```python
from build123d import *

# Parameters (mm, degrees)
F0_R     = 6.35
F1_DEPTH = 12.7
F2_R     = 1.5875
F3_DEPTH = 10.16
F4_W     = 0.4064
F4_H     = 3.728392
F5_DEPTH = 11.4554
F6_SIZE  = 1.27


with BuildPart() as f1:
    # F0 (on Top) → F1 (new body)
    with BuildSketch(Plane.XY):
        Circle(F0_R)
    extrude(amount=-F1_DEPTH)

    # F2 (on face) → F3 (cut)
    with BuildSketch(Plane.XY):
        Circle(F2_R)
    extrude(amount=-F3_DEPTH, mode=Mode.SUBTRACT)

    # F4 (on Top) → F5 (join)
    with BuildSketch(Plane.XY):
        Rectangle(F4_W, F4_H)
    extrude(amount=-F5_DEPTH)

    # F6
    f6_edges = [f1.edges().sort_by_distance(p)[0] for p in [
        (-6.35, 0, -12.7),
    ]]
    chamfer(f6_edges, length=F6_SIZE)


solid = f1.part
```
The model under review builds one solid part; all positions refer to its coordinate system, in mm. A direction names the side the tool comes from. Give positions to 0.01 mm unless a question says otherwise; leave off trailing zeros. Loops run counter-clockwise (first coordinate to the right, second up) from the corner with the lowest first, then second, coordinate; pieces in that order, holes last. Notation, with made-up numbers: (31, -24.5) - (69, -24.5) arc R27 cw to (69, -6.5) - close; hole circle Ø7 at (-28, 67). An arc over 180 degrees is marked (long way). Answer as a JSON object with one key per item and string values.
Q1. Insertion check: pin 1 (3 mm diameter, centred on y = 0.5, z = -9, fed in from +X); pin 2 (1.5 mm diameter, centred on x = 2.5, z = -6, fed in from +Y); pin 3 (2 mm diameter, centred on x = 2.5, z = -9.5, fed in from +Y); pin 4 (2 mm diameter, centred on x = 3, z = -6.5, fed in from +Y). Each pin has a flat end and moves straight along its axis. Give the tip position at first contact, or say it passes through.
Worked out:
{"pin 1": "stops at x = 6.35", "pin 2": "stops at y = 6.1", "pin 3": "stops at y = 6.17", "pin 4": "stops at y = 6.03"}
Q2. Add section C-C on z = -11. State the section outline as (x, y) points.
Worked out:
{"outline": "circle Ø12.7 at (0, 0)"}
Q3. For faces 1 (the flat face through (0.203, 0, -5)), 2 (the flat face through (0, 0, 0)), list the 3-axis set-ups (+Z, -Z, +X, -X, +Y, -Y) from which the entire face can be reached by the end or side of a thin tool; tool diameter is ignored.
Worked out:
{"face 1": "+Z", "face 2": "+Z, +X, -X, +Y, -Y"}
Q4. Mouldability with a two-part tool opening along Y and no side actions: class faces 3 (the cylindrical face through (1.587, -0.032, -5.009)), 4 (the cylindrical face through (-1.38, -6.2, -5.63)), 5 (the flat face through (0, 0, -12.7)) as +Y half, -Y half, draft (parallel to the pull), parting line (faces both ways), or undercut.
Worked out:
{"face 3": "undercut", "face 4": "parting line", "face 5": "draft"}
Q5. Add section A-A on y = 0. State the section outline as (x, z) points, plus the area to 3 significant figures.
Worked out:
{"outline": "(-6.35, -11.43) - (-5.08, -12.7) - (5.08, -12.7) - (6.35, -11.43) - (6.35, 0) - (1.59, 0) - (1.59, -10.16) - (0.2, -10.16) - (0.2, 0) - (-0.2, 0) - (-0.2, -10.16) - (-1.59, -10.16) - (-1.59, 0) - (-6.35, 0) - close", "area": "132 mm^2"}
Q6. Add section B-B on z = -4.5. Count the separate pieces of the cut face and the enclosed holes in it, plus the area to 3 significant figures.
Worked out:
{"separate pieces": "1", "enclosed holes": "2", "area": "120 mm^2"}
Q7. To check wall thickness, follow line 1 along X through (y, z) = (-0.75, -6); line 2 along Y through (x, z) = (1.25, -6); line 3 along Y through (x, z) = (1.75, -11.75). State the ranges of each line that lie inside material, in increasing order.
Worked out:
{"line 1": "x = -6.31 to -1.4, -0.2 to 0.2, 1.4 to 6.31", "line 2": "y = -6.23 to -0.98, 0.98 to 6.23", "line 3": "y = -5.77 to 5.77"}
